Can you work these out from the model? Positions are in its coordinate system, mm. A direction names the side the tool comes from. Give positions to 0.01 mm unless a question says otherwise; leave off trailing zeros. Loops run counter-clockwise (first coordinate to the right, second up) from the corner with the lowest first, then second, coordinate; pieces in that order, holes last. Notation, with made-up numbers: (80, 6.5) -> (133, 6.5) arc R12 ccw to (133, 25.5) -> close; hole circle Ø4 at (-35, -34). An arc over 180 degrees is marked (long way). Return JSON: item names as keys, results as strings. Group by question number.
Q1. Which directions (+Z, -Z, +X, -X, +Y, -Y) give clear straight access to the entire face, cutting with the end or side of a thin tool? Please do faces 5 (the flat face through (0, 0, 12)), 6 (the cylindrical face through (9.902, -77.267, -9.981)).
Q2. Will this pin go through, and if not, where does the flat tip stop? pin 1 (8 mm diameter, centred on x = -7.5, z = -4.5, fed in from +Y).
Q3. Thinking about a two-plate mould opening in Z: for faces 1 (the cylindrical face through (-9.902, -77.267, 9.981)), 2 (the cylindrical face through (-11.251, -77.267, -11.172)), 3 (the cylindrical face through (-11.251, -77.267, 11.172)), 4 (the cylindrical face through (-0.413, -141.327, 12.074)), which applies, pulls with the +Z half, pulls with the -Z half, needs draft (parallel to the pull), parting line crosses it, or undercut?
Q4. Suppose I cut it at A-A, the plane x = 0. Please give me the cut outline in (y, z), and give its area (3 significant figures).
Q5. I need wall thicknesses on line 1 along Y through (x, z) = (0, -12); line 2 along Z through (x, y) = (6.5, -104.5). Which ranges of each line are inside material? Lowest first, please. Write a range as [from, to].
Q6. Suppose I cut it at B-B, the plane y = -85. Please give me the cut outline in (x, z), and give its area (3 significant figures).
Q7. Suppose I cut it at D-D, the plane z = -9.75. Please give me the cut outline in (x, y).
Q8. Suppose I cut it at C-C, the plane z = -1.75. Please give me the cut outline in (x, y).
```python
from build123d import *

# Parameters (mm, degrees)
F0_W     = 25.4
F0_H     = 25.4
F0_W_2   = 22.86
F0_H_2   = 22.86
F1_DEPTH = 152.4
F2_R     = 5.08
F3_R     = 1.857445
F4_DEPTH = 25.401
F6_R     = 3.175
F7_DEPTH = 25.401


with BuildPart() as f1:
    # F0 (on Front) → F1 (new body)
    with BuildSketch(Plane.XZ):
        Rectangle(F0_W, F0_H)
        Rectangle(F0_W_2, F0_H_2, mode=Mode.SUBTRACT)
    extrude(amount=F1_DEPTH)

    # F2
    f2_edges = [f1.edges().sort_by_distance(p)[0] for p in [
        (12.7, -76.2, 12.7),
        (-12.7, -76.2, 12.7),
        (12.7, -76.2, -12.7),
        (-12.7, -76.2, -12.7),
        (11.43, -76.2, 11.43),
        (-11.43, -76.2, 11.43),
        (11.43, -76.2, -11.43),
        (-11.43, -76.2, -11.43),
    ]]
    fillet(f2_edges, radius=F2_R)

    # F3 (on face) → F4 (cut, through all)
    with BuildSketch(Plane.XY.offset(12.7)):
        with Locations((0, -7.9248)):
            Circle(F3_R)
    extrude(amount=-F4_DEPTH, mode=Mode.SUBTRACT)

    # F6 (on face) → F7 (cut, through all)
    with BuildSketch(Plane.XY.offset(12.7)):
        with Locations((0, -144.4752)):
            Circle(F6_R)
    extrude(amount=-F7_DEPTH, mode=Mode.SUBTRACT)


solid = f1.part
```
Ans:
{
 "1": {"face 5": "+Z, -Z, +X, -X, +Y", "face 6": "+Y, -Y"},
 "2": {"pin 1": "stops at y = 0"},
 "3": {"face 1": "undercut", "face 2": "pulls with the -Z half", "face 3": "pulls with the +Z half", "face 4": "needs draft"},
 "4": {"outline": "(-152.4, -12.7) -> (-147.65, -12.7) -> (-147.65, -11.43) -> (-152.4, -11.43) -> close; (-152.4, 11.43) -> (-147.65, 11.43) -> (-147.65, 12.7) -> (-152.4, 12.7) -> close; (-141.3, -12.7) -> (-9.78, -12.7) -> (-9.78, -11.43) -> (-141.3, -11.43) -> close; (-141.3, 11.43) -> (-9.78, 11.43) -> (-9.78, 12.7) -> (-141.3, 12.7) -> close; (-6.07, -12.7) -> (0, -12.7) -> (0, -11.43) -> (-6.07, -11.43) -> close; (-6.07, 11.43) -> (0, 11.43) -> (0, 12.7) -> (-6.07, 12.7) -> close", "area": "362 mm^2"},
 "5": {"line 1": "y = [-152.4, -147.65], [-141.3, -9.78], [-6.07, 0]", "line 2": "z = [-12.7, -11.43], [11.43, 12.7]"},
 "6": {"outline": "(-12.7, -7.62) arc R5.08 ccw to (-7.62, -12.7) -> (7.62, -12.7) arc R5.08 ccw to (12.7, -7.62) -> (12.7, 7.62) arc R5.08 ccw to (7.62, 12.7) -> (-7.62, 12.7) arc R5.08 ccw to (-12.7, 7.62) -> close; hole (-11.43, -6.35) arc R5.08 ccw to (-6.35, -11.43) -> (6.35, -11.43) arc R5.08 ccw to (11.43, -6.35) -> (11.43, 6.35) arc R5.08 ccw to (6.35, 11.43) -> (-6.35, 11.43) arc R5.08 ccw to (-11.43, 6.35) -> close", "area": "123 mm^2"},
 "7": {"outline": "(-12.23, -152.4) -> (-10.12, -152.4) -> (-10.12, 0) -> (-12.23, 0) -> close; (10.12, -152.4) -> (12.23, -152.4) -> (12.23, 0) -> (10.12, 0) -> close"},
 "8": {"outline": "(-12.7, -152.4) -> (-11.43, -152.4) -> (-11.43, 0) -> (-12.7, 0) -> close; (11.43, -152.4) -> (12.7, -152.4) -> (12.7, 0) -> (11.43, 0) -> close"}
}
